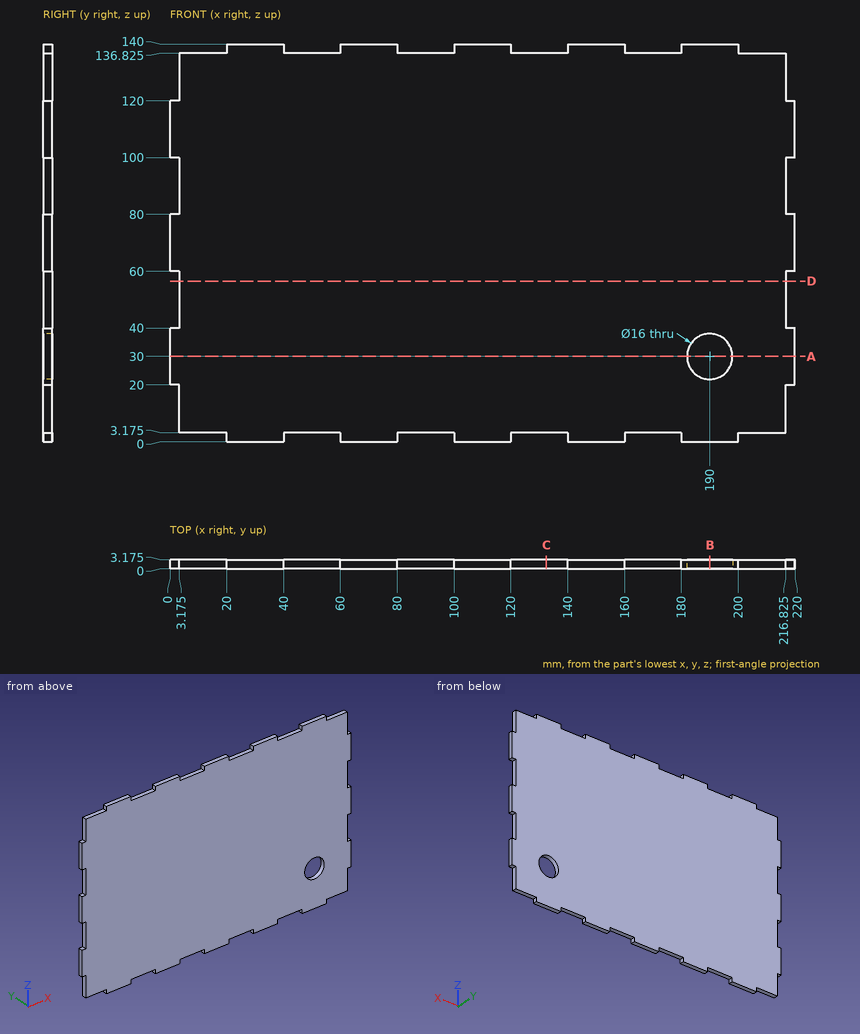
Geometry: see drawing. Coordinates: mm, zero at the bounding-box minimum. Give positions to 0.01 mm unless a question says otherwise; leave off trailing zeros. Order: outer loops, then holes, each group sorted by start corner. A loop starts at its lowest first (then second) coordinate and runs counter-clockwise, first axis right, second up.
Q1. Section C-C on x = 132.5. Output: boundary loops of the cut face in (y, z) (3 decimals), and give its area (3 significant figures).
Checked values:
outline: (0, 3.175) - (3.175, 3.175) - (3.175, 136.825) - (0, 136.825) - close
area: 424 mm2
Q2. Section A-A on z = 30. Output: boundary loops of the cut face in (x, y) (3 decimals), and give its area (3 significant figures).
Checked values:
outline: (0, 0) - (182, 0) - (182, 3.175) - (0, 3.175) - close; (198, 0) - (220, 0) - (220, 3.175) - (198, 3.175) - close
area: 648 mm2
Q3. Ray query, probe 1 along X at (y, z) = (1.1, 30); probe 2 along Z at (x, y) = (190, 2); probe 3 along Z at (x, y) = (175.5, 2.8) (3 decimals). Return the intervals inside material, ascending.
Checked values:
probe 1: x = 0 to 182, 198 to 220
probe 2: z = 0 to 22, 38 to 140
probe 3: z = 3.175 to 136.825
Q4. Section D-D on z = 56.5. Output: boundary loops of the cut face in (x, y) (3 decimals).
Checked values:
outline: (3.175, 0) - (216.825, 0) - (216.825, 3.175) - (3.175, 3.175) - close
Q5. Contact query for flat-ended pins moving along their axis: pin 1 Ø1.6 at (x, y) = (1.5, 2) entering from +Z; pin 2 Ø1 at (y, z) = (1, 138.5) entering from -X; pin 3 Ø1 at (y, z) = (2, 2) entering from +X. Output: stop coordinate, or through.
Checked values:
pin 1: stops at z = 120
pin 2: stops at x = 20
pin 3: stops at x = 200
Q6. Section B-B on x = 190. Output: boundary loops of the cut face in (y, z) (3 decimals), and give its area (3 significant figures).
Checked values:
outline: (0, 0) - (3.175, 0) - (3.175, 22) - (0, 22) - close; (0, 38) - (3.175, 38) - (3.175, 140) - (0, 140) - close
area: 394 mm2
